Part model, mm, in its own coordinate system. A direction names the side the tool comes from. Round coordinates to 2 decimals unless told otherwise and drop trailing zeros. Write each loop counter-clockwise with the first axis right and the second up, starting at its lowest first coordinate (ties: lowest second). Pieces come first, ordered by that corner, then holes. Notation, with made-up numbers: M 24.25,-14.75 L 37.25,-14.75 A27 ccw 37.25,11.25 Z; hole C -23.75,64.25 d11. An arc over 180 degrees is marked long. Use one line per item in the form item = value. Start each with the question number.
Item 1: Cut at B-B, the plane x = 202.25. Give the cut face in (y, z), then the cut area to 3 significant figures.
Item 2: Which spindle directions (+Z, -Z, +X, -X, +Y, -Y) get a long thin tool onto all of the face, cutting with end or side? Do faces 1 (the face through (187, 272, 0)), 2 (the face through (180, 265.897, 1)), 3 (the face through (197, 273.647, 1)). Say none if no direction does.
Item 3: Mould opens along X. For faces 4 (the face through (181.723, 269, 1)), 5 (the face through (188, 264.647, 1)), 6 (the face through (183.56, 282.537, 1.479)), 7 (the face through (180, 272.397, 1)) say: +X half, -X half, draft (parallel to the pull), parting line (faces both ways), or undercut.
Item 4: Cut at C-C, the plane z = 0.3. Give the cut face in (x, y) (3 decimals), then the cut area to 3 significant figures.
Item 5: Cut at A-A, the plane y = 269.5. Give the cut face in (x, z), then the cut area to 3 significant figures.
Item 6: Probe L1, parallel to Y at x = 201, z = 1.5; L2, parallel to X at y = 268.75, z = 1.15; L3, parallel to Y at x = 195.75, z = 0.4. List the from-to ranges inside material, lowest first.
Item 7: Cut at D-D, the plane y = 281.75. Give the cut face in (x, z), then the cut area to 3 significant figures.
Item 8: Flat gauge pins, fed straight in: pin 1 Ø1.5 at (x, z) = (198.5, 2) entering from +Y; pin 2 Ø5 at (x, y) = (201.1, 269.15) entering from +Z. Where does each tip first touch, or does it go through?
from build123d import *

# Parameters (mm, degrees)
MODEL_R                 = 1.5
SALIENTE_EXTRUIR1_DEPTH = 3


with BuildPart() as part:
    # Model → Saliente-Extruir1 (new body)
    with BuildSketch(Plane.XY):
        with BuildLine():
            Line((182.972853309, 282.646547335), (175.597853309, 282.646547335))
            Line((175.597853309, 282.646547335), (175.597853309, 264.646547335))
            Line((175.597853309, 264.646547335), (201.097853309, 264.646547335))
            ThreePointArc((201.097853309, 264.646547335), (205.597853309, 269.146547335), (201.097853309, 273.646547335))
            Line((201.097853309, 273.646547335), (193.660353309, 273.646547335))
            Line((193.660353309, 273.646547335), (184.055904605, 282.233003026))
            ThreePointArc((184.055904605, 282.233003026), (183.552512477, 282.539644911), (182.972853309, 282.646547335))
        make_face()
        with Locations((201.097853309, 269.146547335)):
            Circle(MODEL_R, mode=Mode.SUBTRACT)
        with Locations((180.097853309, 278.145968764)):
            Circle(MODEL_R, mode=Mode.SUBTRACT)
        with BuildLine():
            Line((179.222853309, 265.896547335), (180.972853309, 265.896547335))
            ThreePointArc((180.972853309, 265.896547335), (181.503183395, 266.116217249), (181.722853309, 266.646547335))
            Line((181.722853309, 266.646547335), (181.722853309, 271.646547335))
            ThreePointArc((181.722853309, 271.646547335), (181.503183395, 272.176877421), (180.972853309, 272.396547335))
            Line((180.972853309, 272.396547335), (179.222853309, 272.396547335))
            ThreePointArc((179.222853309, 272.396547335), (178.692523223, 272.176877421), (178.472853309, 271.646547335))
            Line((178.472853309, 271.646547335), (178.472853309, 266.646547335))
            ThreePointArc((178.472853309, 266.646547335), (178.692523223, 266.116217249), (179.222853309, 265.896547335))
        make_face(mode=Mode.SUBTRACT)
    extrude(amount=SALIENTE_EXTRUIR1_DEPTH)


solid = part.part
Model answer:
q1.outline = M 264.8,0 L 268.19,0 L 268.19,3 L 264.8,3 Z; M 270.11,0 L 273.5,0 L 273.5,3 L 270.11,3 Z
q1.area = 20.3 mm²
q2.face_1 = -Z, +X, -X, +Y, -Y
q2.face_2 = +Z, -Z
q2.face_3 = +Z, -Z, +X, +Y
q3.face_4 = undercut
q3.face_5 = draft
q3.face_6 = +X half
q3.face_7 = undercut
q4.outline = M 175.598,264.647 L 201.098,264.647 A4.5 ccw 201.098,273.647 L 193.66,273.647 L 184.056,282.233 A1.625 ccw 182.973,282.647 L 175.598,282.647 Z; hole M 178.473,266.647 A0.75 ccw 179.223,265.897 L 180.973,265.897 A0.75 ccw 181.723,266.647 L 181.723,271.647 A0.75 ccw 180.973,272.397 L 179.223,272.397 A0.75 ccw 178.473,271.647 Z; hole C 180.098,278.146 d3; hole C 201.098,269.147 d3
q4.area = 344 mm²
q5.outline = M 175.6,0 L 178.47,0 L 178.47,3 L 175.6,3 Z; M 181.72,0 L 199.64,0 L 199.64,3 L 181.72,3 Z; M 202.56,0 L 205.58,0 L 205.58,3 L 202.56,3 Z
q5.area = 71.5 mm²
q6.L1 = 264.65 to 267.65, 270.64 to 273.65
q6.L2 = 175.6 to 178.47, 181.72 to 199.65, 202.54 to 205.58
q6.L3 = 264.65 to 273.65
q7.outline = M 175.6,0 L 184.6,0 L 184.6,3 L 175.6,3 Z
q7.area = 27.0 mm²
q8.pin_1 = 273.65
q8.pin_2 = 3
